```python
from build123d import *

# Parameters (mm, degrees)
SKETCH1_W                 = 50.8
SKETCH1_H                 = 25.4
BASE_DEPTH                = 2.54
SKETCH2_R                 = 1.27
GUIDEPOSTS_DEPTH          = 12.7
SKETCH3_W                 = 17.78
SKETCH3_H                 = 2.54
BUTTON_HOLDER_DEPTH       = 15.24
ROUND_ON_BUTTON_HOLDER_R  = 2.54
ONE_BUTTON_LEG_HOLE_REACH = 40.556
BUTTON_LEG_HOLES_COUNT    = 4


with BuildPart() as part:
    # Sketch1 → base (new body)
    with BuildSketch(Plane.XY):
        Rectangle(SKETCH1_W, SKETCH1_H)
    extrude(amount=BASE_DEPTH)

    # Sketch2 → guideposts (add)
    with BuildSketch(Plane.XY.offset(2.54)):
        with Locations(Location((7.590347968, -1.846813132, 0), (0, 0, 180))):
            Circle(SKETCH2_R)
        with Locations(Location((7.590347968, -5.285256746, 0), (0, 0, 180))):
            Circle(SKETCH2_R)
        with Locations(Location((-13.597624432, -3.751813132, 0), (0, 0, 180))):
            Circle(SKETCH2_R)
    extrude(amount=GUIDEPOSTS_DEPTH)

    # Sketch3 → button holder (add)
    with BuildSketch(Plane.XY.offset(2.54)):
        with Locations((-14.105624432, 8.948186868)):
            Rectangle(SKETCH3_W, SKETCH3_H)
    extrude(amount=BUTTON_HOLDER_DEPTH)

    # round on button holder
    # the kernel refuses this fillet: 2.54 mm, written as the material it adds along each edge
    with BuildSketch(Plane(origin=(7.590347968, -1.846813132, 2.54), x_dir=(-1, 0, 0), z_dir=(0, 1, 0))) as round_on_button_holder_piece_1:
        with BuildLine():
            CenterArc((1.27 + ROUND_ON_BUTTON_HOLDER_R, ROUND_ON_BUTTON_HOLDER_R), ROUND_ON_BUTTON_HOLDER_R, 180, 90)
            Line((1.27, ROUND_ON_BUTTON_HOLDER_R), (1.27, 0))
            Line((1.27, 0), (1.27 + ROUND_ON_BUTTON_HOLDER_R, 0))
        make_face()
    round_on_button_holder_piece_1_solid = revolve(axis=Axis((7.590347968, -1.846813132, 2.54), (0, 0, 1)), mode=Mode.PRIVATE)
    with BuildSketch(Plane(origin=(7.590347968, -5.285256746, 2.54), x_dir=(-1, 0, 0), z_dir=(0, 1, 0))) as round_on_button_holder_piece_2:
        with BuildLine():
            CenterArc((1.27 + ROUND_ON_BUTTON_HOLDER_R, ROUND_ON_BUTTON_HOLDER_R), ROUND_ON_BUTTON_HOLDER_R, 180, 90)
            Line((1.27, ROUND_ON_BUTTON_HOLDER_R), (1.27, 0))
            Line((1.27, 0), (1.27 + ROUND_ON_BUTTON_HOLDER_R, 0))
        make_face()
    round_on_button_holder_piece_2_solid = revolve(axis=Axis((7.590347968, -5.285256746, 2.54), (0, 0, 1)), mode=Mode.PRIVATE)
    with BuildSketch(Plane(origin=(-13.597624432, -3.751813132, 2.54), x_dir=(-1, 0, 0), z_dir=(0, 1, 0))) as round_on_button_holder_piece_3:
        with BuildLine():
            CenterArc((1.27 + ROUND_ON_BUTTON_HOLDER_R, ROUND_ON_BUTTON_HOLDER_R), ROUND_ON_BUTTON_HOLDER_R, 180, 90)
            Line((1.27, ROUND_ON_BUTTON_HOLDER_R), (1.27, 0))
            Line((1.27, 0), (1.27 + ROUND_ON_BUTTON_HOLDER_R, 0))
        make_face()
    round_on_button_holder_piece_3_solid = revolve(axis=Axis((-13.597624432, -3.751813132, 2.54), (0, 0, 1)), mode=Mode.PRIVATE)
    with BuildSketch(Plane(origin=(-5.215624432, 7.678186868, 2.54), x_dir=(1, 0, 0), z_dir=(0, 1, 0))) as round_on_button_holder_piece_4:
        with BuildLine():
            CenterArc((ROUND_ON_BUTTON_HOLDER_R, -ROUND_ON_BUTTON_HOLDER_R), ROUND_ON_BUTTON_HOLDER_R, 90, 90)
            Line((0, -ROUND_ON_BUTTON_HOLDER_R), (0, 0))
            Line((0, 0), (ROUND_ON_BUTTON_HOLDER_R, 0))
        make_face()
    round_on_button_holder_piece_4_solid = extrude(amount=2.54, mode=Mode.PRIVATE)
    with BuildSketch(Plane(origin=(-5.215624432, 10.218186868, 2.54), x_dir=(0, 1, 0), z_dir=(-1, 0, 0))) as round_on_button_holder_piece_5_section:
        with BuildLine():
            CenterArc((ROUND_ON_BUTTON_HOLDER_R, -ROUND_ON_BUTTON_HOLDER_R), ROUND_ON_BUTTON_HOLDER_R, 90, 90)
            Line((0, -ROUND_ON_BUTTON_HOLDER_R), (0, 0))
            Line((0, 0), (ROUND_ON_BUTTON_HOLDER_R, 0))
        make_face()
    round_on_button_holder_piece_5 = extrude(amount=17.78, mode=Mode.PRIVATE)
    round_on_button_holder_piece_5 = split(round_on_button_holder_piece_5, bisect_by=Plane(origin=(-5.215624432, 12.7, 2.54), z_dir=(0, -1, 0)), keep=Keep.TOP, mode=Mode.PRIVATE)
    with BuildSketch(Plane(origin=(-22.995624432, 10.218186868, 2.54), x_dir=(-1, 0, 0), z_dir=(0, -1, 0))) as round_on_button_holder_piece_6:
        with BuildLine():
            CenterArc((2.54, -2.536376552), ROUND_ON_BUTTON_HOLDER_R, 93.060789284, 86.939210716)
            Line((0, -2.536376552), (0, 0))
            Line((0, 0), (2.404375568, 0))
        make_face()
    round_on_button_holder_piece_6_solid = extrude(amount=2.54, mode=Mode.PRIVATE)
    with BuildSketch(Plane(origin=(-22.995624432, 7.678186868, 2.54), x_dir=(0, -1, 0), z_dir=(1, 0, 0))) as round_on_button_holder_piece_7:
        with BuildLine():
            CenterArc((ROUND_ON_BUTTON_HOLDER_R, -ROUND_ON_BUTTON_HOLDER_R), ROUND_ON_BUTTON_HOLDER_R, 90, 90)
            Line((0, -ROUND_ON_BUTTON_HOLDER_R), (0, 0))
            Line((0, 0), (ROUND_ON_BUTTON_HOLDER_R, 0))
        make_face()
    round_on_button_holder_piece_7_solid = extrude(amount=17.78, mode=Mode.PRIVATE)
    with BuildSketch(Plane(origin=(-22.995624432, 7.678186868, 2.54), x_dir=(0, -1, 0), z_dir=(1, 0, 0))) as round_on_button_holder_piece_8a_section:
        with BuildLine():
            CenterArc((ROUND_ON_BUTTON_HOLDER_R, -ROUND_ON_BUTTON_HOLDER_R), ROUND_ON_BUTTON_HOLDER_R, 90, 90)
            Line((0, -ROUND_ON_BUTTON_HOLDER_R), (0, 0))
            Line((0, 0), (ROUND_ON_BUTTON_HOLDER_R, 0))
        make_face()
    round_on_button_holder_piece_8a = extrude(amount=24.13, mode=Mode.PRIVATE)
    round_on_button_holder_piece_8a = split(round_on_button_holder_piece_8a, bisect_by=Plane(origin=(-5.215624432, 7.678186868, 2.54), z_dir=(1, 0, 0)), keep=Keep.TOP, mode=Mode.PRIVATE)
    with BuildSketch(Plane(origin=(-5.215624432, 1.328186868, 2.54), x_dir=(1, 0, 0), z_dir=(0, 1, 0))) as round_on_button_holder_piece_8b_section:
        with BuildLine():
            CenterArc((ROUND_ON_BUTTON_HOLDER_R, -ROUND_ON_BUTTON_HOLDER_R), ROUND_ON_BUTTON_HOLDER_R, 90, 90)
            Line((0, -ROUND_ON_BUTTON_HOLDER_R), (0, 0))
            Line((0, 0), (ROUND_ON_BUTTON_HOLDER_R, 0))
        make_face()
    round_on_button_holder_piece_8b = extrude(amount=8.89, mode=Mode.PRIVATE)
    round_on_button_holder_piece_8b = split(round_on_button_holder_piece_8b, bisect_by=Plane(origin=(-5.215624432, 7.678186868, 2.54), z_dir=(0, -1, 0)), keep=Keep.TOP, mode=Mode.PRIVATE)
    round_on_button_holder_piece_8 = round_on_button_holder_piece_8a & round_on_button_holder_piece_8b
    with BuildSketch(Plane(origin=(-5.215624432, 7.678186868, 2.54), x_dir=(1, 0, 0), z_dir=(0, 1, 0))) as round_on_button_holder_piece_9a_section:
        with BuildLine():
            CenterArc((ROUND_ON_BUTTON_HOLDER_R, -ROUND_ON_BUTTON_HOLDER_R), ROUND_ON_BUTTON_HOLDER_R, 90, 90)
            Line((0, -ROUND_ON_BUTTON_HOLDER_R), (0, 0))
            Line((0, 0), (ROUND_ON_BUTTON_HOLDER_R, 0))
        make_face()
    round_on_button_holder_piece_9a = extrude(amount=8.89, mode=Mode.PRIVATE)
    round_on_button_holder_piece_9a = split(round_on_button_holder_piece_9a, bisect_by=Plane(origin=(-5.215624432, 12.7, 2.54), z_dir=(0, -1, 0)), keep=Keep.TOP, mode=Mode.PRIVATE)
    round_on_button_holder_piece_9a = split(round_on_button_holder_piece_9a, bisect_by=Plane(origin=(-5.215624432, 10.218186868, 2.54), z_dir=(0, 1, 0)), keep=Keep.TOP, mode=Mode.PRIVATE)
    with BuildSketch(Plane(origin=(1.134375568, 10.218186868, 2.54), x_dir=(0, 1, 0), z_dir=(-1, 0, 0))) as round_on_button_holder_piece_9b_section:
        with BuildLine():
            CenterArc((ROUND_ON_BUTTON_HOLDER_R, -ROUND_ON_BUTTON_HOLDER_R), ROUND_ON_BUTTON_HOLDER_R, 90, 90)
            Line((0, -ROUND_ON_BUTTON_HOLDER_R), (0, 0))
            Line((0, 0), (ROUND_ON_BUTTON_HOLDER_R, 0))
        make_face()
    round_on_button_holder_piece_9b = extrude(amount=24.13, mode=Mode.PRIVATE)
    round_on_button_holder_piece_9b = split(round_on_button_holder_piece_9b, bisect_by=Plane(origin=(-5.215624432, 10.218186868, 2.54), z_dir=(1, 0, 0)), keep=Keep.TOP, mode=Mode.PRIVATE)
    round_on_button_holder_piece_9 = round_on_button_holder_piece_9a & round_on_button_holder_piece_9b
    with BuildSketch(Plane(origin=(-5.215624432, 10.218186868, 2.54), x_dir=(0, 1, 0), z_dir=(-1, 0, 0))) as round_on_button_holder_piece_10a_section:
        with BuildLine():
            CenterArc((ROUND_ON_BUTTON_HOLDER_R, -ROUND_ON_BUTTON_HOLDER_R), ROUND_ON_BUTTON_HOLDER_R, 90, 90)
            Line((0, -ROUND_ON_BUTTON_HOLDER_R), (0, 0))
            Line((0, 0), (ROUND_ON_BUTTON_HOLDER_R, 0))
        make_face()
    round_on_button_holder_piece_10a = extrude(amount=24.13, mode=Mode.PRIVATE)
    round_on_button_holder_piece_10a = split(round_on_button_holder_piece_10a, bisect_by=Plane(origin=(-25.4, 10.218186868, 2.54), z_dir=(1, 0, 0)), keep=Keep.TOP, mode=Mode.PRIVATE)
    round_on_button_holder_piece_10a = split(round_on_button_holder_piece_10a, bisect_by=Plane(origin=(-22.995624432, 10.218186868, 2.54), z_dir=(-1, 0, 0)), keep=Keep.TOP, mode=Mode.PRIVATE)
    with BuildSketch(Plane(origin=(-22.995624432, 16.559128248, 2.54), x_dir=(-1, 0, 0), z_dir=(0, -1, 0))) as round_on_button_holder_piece_10b_section:
        with BuildLine():
            CenterArc((2.54, -2.536376552), ROUND_ON_BUTTON_HOLDER_R, 93.060789284, 86.939210716)
            Line((0, -2.536376552), (0, 0))
            Line((0, 0), (2.404375568, 0))
        make_face()
    round_on_button_holder_piece_10b = extrude(amount=8.88094138, mode=Mode.PRIVATE)
    round_on_button_holder_piece_10b = split(round_on_button_holder_piece_10b, bisect_by=Plane(origin=(-22.995624432, 12.7, 2.54), z_dir=(0, -1, 0)), keep=Keep.TOP, mode=Mode.PRIVATE)
    round_on_button_holder_piece_10b = split(round_on_button_holder_piece_10b, bisect_by=Plane(origin=(-22.995624432, 10.218186868, 2.54), z_dir=(0, 1, 0)), keep=Keep.TOP, mode=Mode.PRIVATE)
    round_on_button_holder_piece_10 = round_on_button_holder_piece_10a & round_on_button_holder_piece_10b
    with BuildSketch(Plane(origin=(-29.345624432, 7.678186868, 2.54), x_dir=(0, -1, 0), z_dir=(1, 0, 0))) as round_on_button_holder_piece_11a_section:
        with BuildLine():
            CenterArc((ROUND_ON_BUTTON_HOLDER_R, -ROUND_ON_BUTTON_HOLDER_R), ROUND_ON_BUTTON_HOLDER_R, 90, 90)
            Line((0, -ROUND_ON_BUTTON_HOLDER_R), (0, 0))
            Line((0, 0), (ROUND_ON_BUTTON_HOLDER_R, 0))
        make_face()
    round_on_button_holder_piece_11a = extrude(amount=24.13, mode=Mode.PRIVATE)
    round_on_button_holder_piece_11a = split(round_on_button_holder_piece_11a, bisect_by=Plane(origin=(-25.4, 7.678186868, 2.54), z_dir=(1, 0, 0)), keep=Keep.TOP, mode=Mode.PRIVATE)
    round_on_button_holder_piece_11a = split(round_on_button_holder_piece_11a, bisect_by=Plane(origin=(-22.995624432, 7.678186868, 2.54), z_dir=(-1, 0, 0)), keep=Keep.TOP, mode=Mode.PRIVATE)
    with BuildSketch(Plane(origin=(-22.995624432, 10.218186868, 2.54), x_dir=(-1, 0, 0), z_dir=(0, -1, 0))) as round_on_button_holder_piece_11b_section:
        with BuildLine():
            CenterArc((2.54, -2.536376552), ROUND_ON_BUTTON_HOLDER_R, 93.060789284, 86.939210716)
            Line((0, -2.536376552), (0, 0))
            Line((0, 0), (2.404375568, 0))
        make_face()
    round_on_button_holder_piece_11b = extrude(amount=8.88094138, mode=Mode.PRIVATE)
    round_on_button_holder_piece_11b = split(round_on_button_holder_piece_11b, bisect_by=Plane(origin=(-22.995624432, 7.678186868, 2.54), z_dir=(0, -1, 0)), keep=Keep.TOP, mode=Mode.PRIVATE)
    round_on_button_holder_piece_11 = round_on_button_holder_piece_11a & round_on_button_holder_piece_11b
    add([round_on_button_holder_piece_1_solid, round_on_button_holder_piece_2_solid, round_on_button_holder_piece_3_solid, round_on_button_holder_piece_4_solid, round_on_button_holder_piece_5, round_on_button_holder_piece_6_solid, round_on_button_holder_piece_7_solid, round_on_button_holder_piece_8, round_on_button_holder_piece_9, round_on_button_holder_piece_10, round_on_button_holder_piece_11])

    # Sketch4 → one button leg hole (cut, up to next)
    with BuildSketch(Plane(origin=(0, 10.218186868, 0), x_dir=(1, 0, 0), z_dir=(0, 1, 0)), mode=Mode.PRIVATE) as one_button_leg_hole_sk1:
        with BuildLine():
            Line((-15.121624432, -14.224), (-13.089624432, -14.224))
            ThreePointArc((-13.089624432, -14.224), (-12.073624432, -15.24), (-13.089624432, -16.256))
            Line((-13.089624432, -16.256), (-15.121624432, -16.256))
            ThreePointArc((-15.121624432, -16.256), (-16.137624432, -15.24), (-15.121624432, -14.224))
        make_face()
    one_button_leg_hole_tool1 = extrude(one_button_leg_hole_sk1.sketch, amount=-ONE_BUTTON_LEG_HOLE_REACH, mode=Mode.PRIVATE) & part.part
    one_button_leg_hole = one_button_leg_hole_tool1.solids().sort_by_distance((-14.105624, 10.218187, 15.24))[0]
    add(one_button_leg_hole, mode=Mode.SUBTRACT)

    # button leg holes: one button leg hole ×4 about axis
    button_leg_holes_axis = Axis((-14.105624476, 0, 11.429666717), (0, 1, 0))
    for i in range(1, BUTTON_LEG_HOLES_COUNT):
        add(one_button_leg_hole.rotate(button_leg_holes_axis, i * 360 / BUTTON_LEG_HOLES_COUNT), mode=Mode.SUBTRACT)


solid = part.part
```
Can you work these out from the model? Positions are in its coordinate system, mm. A direction names the side the tool comes from. Round coordinates to 2 decimals unless told otherwise and drop trailing zeros. Loops run counter-clockwise (first coordinate to the right, second up) from the corner with the lowest first, then second, coordinate; pieces in that order, holes last. Notation, with made-up numbers: (47, -26) -> (100, -26) arc R26 ccw to (100, -2) -> close; hole circle Ø9 at (47.25, 4). An arc over 180 degrees is marked (long way). One line per item, written item: value. Start each with the question number.
1. For pin 1 (10 mm diameter, centred on y = -10, z = 16, fed in from -X); pin 2 (2 mm diameter, centred on y = 9, z = 12, fed in from +X); pin 3 (5 mm diameter, centred on x = 2.5, y = -4, fed in from +Z); pin 4 (1 mm diameter, centred on y = -9, z = 4.5, fed in from -X), each with a flat end and sliding along its axis, tell me the tip position at first contact or that it passes through.
2. If I drill on probe 1 along Z at (x, y) = (14, -4.5); probe 2 along Z at (x, y) = (-14.5, -3.25); probe 3 along Y at (x, z) = (-8.5, 7.25), over which ranges is the centre line in solid material (lowest first)?
3. If we section it at C-C, the plane x = 12.5: Write out the boundary of the cut face in (y, z).
4. If we mould it in two halves opening along Z, with no side actions, what happens to faces 1 (the cylindrical face through (-10.27, 8.97, 13.46)), 2 (the flat face through (0, 0, 0)), 3 (the cylindrical face through (8.598, -1.074, 10.089))? For each: pulls with the +Z half, pulls with the -Z half, needs draft (parallel to the pull), parting line crosses it, or undercut.
5. For faces 4 (the flat face through (-14, 9, 8.635)), 5 (the cylindrical face through (-17.89, 8.97, 13.46)), 6 (the flat face through (0, 0, 2.54)), 7 (the flat face through (-22.996, 9, 11)), which set-ups out of +Z, -Z, +X, -X, +Y, -Y let a thin tool reach every point of the face, with its end or its side?
6. If we section it at A-A, the plane z = 3.5: Write out the boundary of the cut face in (x, y).
7. If we section it at D-D, the plane y = 4.5: Write out the boundary of the cut face in (x, z), then the cut area to 3 significant figures.
8. If we section it at B-B, the plane y = 11.25: Write out the boundary of the cut face in (x, z).
Calculated:
1. pin 1: stops at x = 6.32
1. pin 2: stops at x = -5.22
1. pin 3: stops at z = 2.77
1. pin 4: passes through
2. probe 1: z = 0 to 2.54
2. probe 2: z = 0 to 15.24
2. probe 3: y = 7.68 to 10.22
3. outline: (-12.7, 0) -> (12.7, 0) -> (12.7, 2.54) -> (-12.7, 2.54) -> close
4. face 1: undercut
4. face 2: pulls with the -Z half
4. face 3: needs draft
5. face 4: +Y
5. face 5: +Y, -Y
5. face 6: +Z
5. face 7: +Z, -X, +Y, -Y
6. outline: (-23.54, 7.13) -> (-4.66, 7.13) -> (-4.66, 10.77) -> (-23.54, 10.77) -> close; circle Ø3.64 at (-13.6, -3.75); (6.99, -3.57) arc R1.82 ccw (long way) to (8.19, -3.57) arc R1.82 ccw (long way) to start
7. outline: (-25.4, 0) -> (25.4, 0) -> (25.4, 2.54) -> (-25.4, 2.54) -> close
7. area: 129 mm²
8. outline: (-25.4, 0) -> (25.4, 0) -> (25.4, 2.54) -> (-2.68, 2.54) arc R2.54 cw to (-4.18, 3.04) -> (-24.02, 3.04) arc R2.54 cw to (-25.4, 2.54) -> close
